CAD build for the part. Positions are in the model's coordinates, mm. A direction names the side the tool comes from. Give positions to 0.01 mm unless a question says otherwise; leave off trailing zeros. Loops run counter-clockwise (first coordinate to the right, second up) from the corner with the lowest first, then second, coordinate; pieces in that order, holes last. Notation, with made-up numbers: (-2.75, -18) -> (30.25, -18) arc R31 ccw to (30.25, 8) -> close; hole circle Ø11 at (64, -27.5). An arc over 180 degrees is marked (long way). Use one line per item in the form item = value.
```python
from build123d import *

# Parameters (mm, degrees)
SKETCH_W        = 57
SKETCH_H        = 30
PAD_DEPTH       = 13
SKETCH001_W     = 53
SKETCH001_H     = 26
POCKET_DEPTH    = 11
SKETCH002_R     = 1
POCKET001_DEPTH = 2.001


with BuildPart() as part:
    # Sketch → Pad (new body)
    with BuildSketch(Plane.XY):
        with Locations((0, 15)):
            Rectangle(SKETCH_W, SKETCH_H)
    extrude(amount=PAD_DEPTH)

    # Sketch001 (on Face6 of Pad) → Pocket (cut)
    with BuildSketch(Plane.XY.offset(13)):
        with Locations((0, 15)):
            Rectangle(SKETCH001_W, SKETCH001_H)
    extrude(amount=-POCKET_DEPTH, mode=Mode.SUBTRACT)

    # Sketch002 (on Face11 of Pocket) → Pocket001 (cut, through all)
    with BuildSketch(Plane.XY.offset(2)):
        with Locations((0, 22.5)):
            Circle(SKETCH002_R)
        with Locations((0, 7.5)):
            Circle(SKETCH002_R)
    extrude(amount=-POCKET001_DEPTH, mode=Mode.SUBTRACT)


solid = part.part
```
1. Cut at A-A, the plane y = 22.5. Write the cut outline in (x, z), then the cut area to 3 significant figures.
Result sheet:
outline = (-28.5, 0) -> (-1, 0) -> (-1, 2) -> (-26.5, 2) -> (-26.5, 13) -> (-28.5, 13) -> close; (1, 0) -> (28.5, 0) -> (28.5, 13) -> (26.5, 13) -> (26.5, 2) -> (1, 2) -> close
area = 154 mm^2
2. Cut at D-D, the plane y = 13.25. Write the cut outline in (x, z).
Result sheet:
outline = (-28.5, 0) -> (28.5, 0) -> (28.5, 13) -> (26.5, 13) -> (26.5, 2) -> (-26.5, 2) -> (-26.5, 13) -> (-28.5, 13) -> close
3. Mould opens along X. For faces 3 (the flat face through (28.5, 15, 6)), 4 (the flat face through (0, 28, 8)), 5 (the flat face through (-26.5, 15, 8)), 6 (the flat face through (0, 15, 0)) say: pulls with the +X half, pulls with the -X half, needs draft (parallel to the pull), parting line crosses it, or undercut.
Result sheet:
face_3 = pulls with the +X half
face_4 = undercut
face_5 = undercut
face_6 = needs draft
4. Cut at B-B, the plane x = 0. Write the cut outline in (y, z).
Result sheet:
outline = (0, 0) -> (6.5, 0) -> (6.5, 2) -> (2, 2) -> (2, 13) -> (0, 13) -> close; (8.5, 0) -> (21.5, 0) -> (21.5, 2) -> (8.5, 2) -> close; (23.5, 0) -> (30, 0) -> (30, 13) -> (28, 13) -> (28, 2) -> (23.5, 2) -> close
5. Drop a flat-ended pin along its axis: P1, Ø2.5, axis at x = 0, y = 7.5, coming from the +Z side. Give the stop position or say it passes through.
Result sheet:
P1 = 2
6. Tool access for faces 1 (the flat face through (0, 30, 6)), 2 (the flat face through (0, 15, 2)): list every direction of +Z, -Z, +X, -X, +Y, -Y with a clear straight run to the whole face (end or side of a thin tool).
Result sheet:
face_1 = +Z, -Z, +X, -X, +Y
face_2 = +Z
7. Drill centre lines: line 1 (Y direction, x = 0, z = 1.35); line 2 (Y direction, x = 24.5, z = 8); line 3 (X direction, y = 20.25, z = 12.5). Where is each one in solid material? Low to high.
Result sheet:
line_1 = 0 to 6.5, 8.5 to 21.5, 23.5 to 30
line_2 = 0 to 2, 28 to 30
line_3 = -28.5 to -26.5, 26.5 to 28.5
8. Cut at C-C, the plane z = 2.75. Write the cut outline in (x, y), then the cut area to 3 significant figures.
Result sheet:
outline = (-28.5, 0) -> (28.5, 0) -> (28.5, 30) -> (-28.5, 30) -> close; hole (-26.5, 2) -> (26.5, 2) -> (26.5, 28) -> (-26.5, 28) -> close
area = 332 mm^2
